Can you work these out from the drawing? Everything is in mm from the part's minimum corner. A direction names the side the tool comes from. Give positions to 0.01 mm unless a question says otherwise; leave off trailing zeros. Write each loop counter-clockwise with the first axis right and the second up, starting at its lowest first coordinate (ties: lowest second). Pieces come first, ordered by that corner, then holes. Notation, with made-up numbers: (-26, -25.5) - (-21, -25.5) arc R31 ccw to (-21, 3.5) - close; hole circle Ø3 at (16.5, -27.5). An arc over 180 degrees is marked (long way). Write each question's results on one line, items separated by ' | '. Start each with the question number.
Item 1: Suppose I cut it at B-B on z = 22.25. List the corners of the cut face in (x, y) for me.
Item 2: Suppose I cut it at A-A on x = 24. List the corners of the cut face in (y, z) for me, then the cut area to 3 significant figures.
Item 3: Which directions (+Z, -Z, +X, -X, +Y, -Y) give clear straight access to the entire face, cutting with the end or side of a thin tool? Please do the marked faces 1, 2, 3 and 4.
Item 4: Suppose I cut it at C-C on y = 17.5. List the corners of the cut face in (x, z) for me.
Item 5: Please list where these lines run through material, in increasing order: line 1 along X through (y, z) = (14.5, 23.5); line 2 along Y through (x, z) = (23, 22.25); line 3 along Z through (x, y) = (26, 26).
Item 6: Will these pins go through, and if not, where does the flat tip stop? P1, Ø5, axis at x = 30, z = 17.5, coming from the -Y side; P2, Ø4, axis at x = 5, y = 9.5, coming from the -Z side (3 decimals); P3, Ø4.5, axis at x = 20.5, y = 15, coming from the +Z side; P4, Ø2, axis at y = 17.5, z = 24.5, coming from the +X side.
Item 7: Suppose I cut it at D-D on z = 17.25. List the corners of the cut face in (x, y) for me, then the cut area to 3 significant figures.
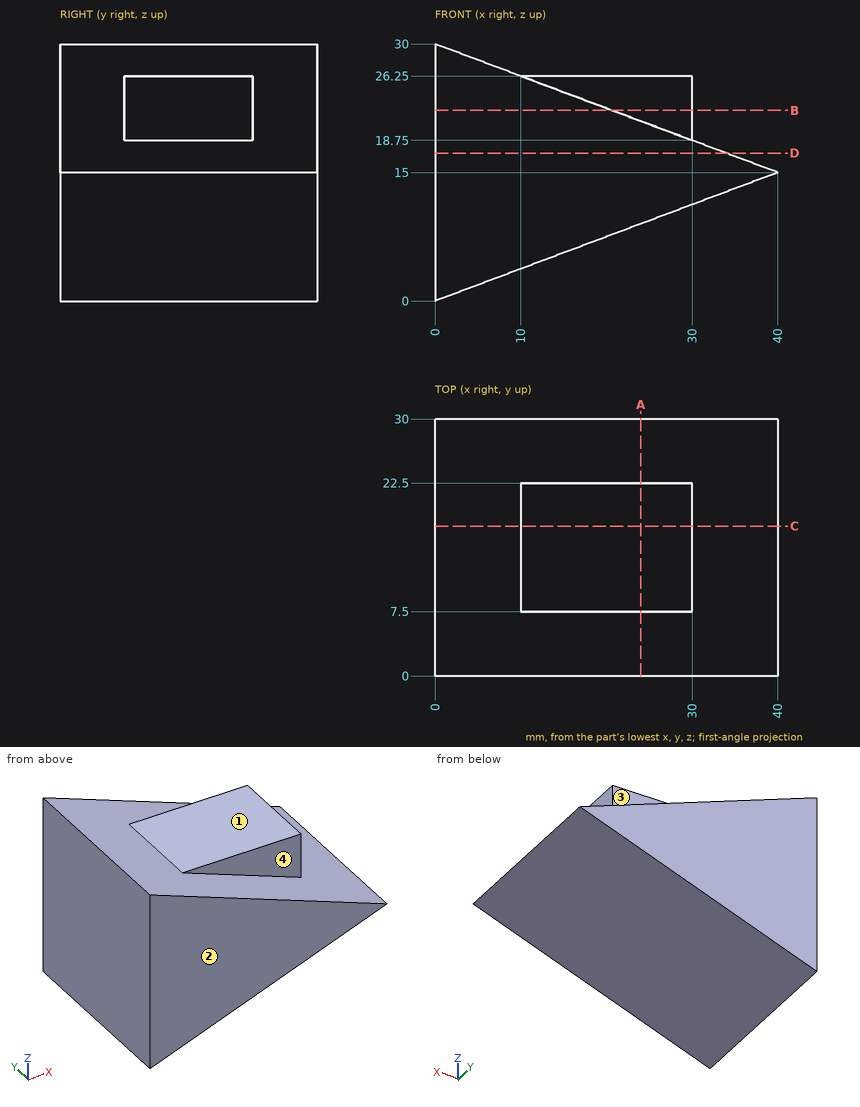
Checked values:
1) outline: (0, 0) - (20.67, 0) - (20.67, 7.5) - (30, 7.5) - (30, 22.5) - (20.67, 22.5) - (20.67, 30) - (0, 30) - close
2) outline: (0, 9) - (30, 9) - (30, 21) - (22.5, 21) - (22.5, 26.25) - (7.5, 26.25) - (7.5, 21) - (0, 21) - close | area: 439 mm^2
3) face 1: +Z, +X, +Y, -Y | face 2: +Z, -Z, +X, -X, -Y | face 3: +Z, +X, +Y | face 4: +Z, +X, -Y
4) outline: (0, 0) - (40, 15) - (30, 18.75) - (30, 26.25) - (10, 26.25) - (0, 30) - close
5) line 1: x = 0 to 30 | line 2: y = 7.5 to 22.5 | line 3: z = 9.75 to 20.25
6) P1: stops at y = 0 | P2: stops at z = 1.125 | P3: stops at z = 26.25 | P4: stops at x = 30
7) outline: (0, 0) - (34, 0) - (34, 30) - (0, 30) - close | area: 1,020 mm^2
